Could you check a few things on this model? Use its own coordinates, in mm. A direction names the side the tool comes from. Round coordinates to 2 decimals unless told otherwise and drop trailing zeros. Write each loop counter-clockwise with the first axis right and the second up, starting at its lowest first coordinate (ties: lowest second). Pieces come first, ordered by that corner, then holes. Notation, with made-up numbers: (-35.75, 28.5) -> (9.25, 28.5) arc R14 cw to (9.25, 44.5) -> close; hole circle Ø6 at (-5.75, 34.25). An arc over 180 degrees is marked (long way). Answer in a Markdown table with one row per item.
from build123d import *

# Parameters (mm, degrees)
BOSS_EXTRUDE1_DEPTH      = 1.5
BOSS_EXTRUDE1_DEPTH_BACK = 1.5
SKETCH1_R                = 5
SKETCH1_R_2              = 2
FILLET1_R                = 100
SKETCH2_R                = 1.5
CUT_EXTRUDE1_DEPTH       = 10


with BuildPart() as part:
    # Sketch1 → Boss-Extrude1 (new, two sides: drawn at the far end of the back side and taken through both)
    with BuildSketch(Plane(origin=(0, 0, 0), x_dir=(1, 0, 0), z_dir=(0, 1, 0)).offset(-BOSS_EXTRUDE1_DEPTH_BACK)):
        with BuildLine():
            Line((0, 15), (-139.784941349, 43.225909045))
            Line((-139.784941349, 43.225909045), (-351.875415017, 29.941322925))
            ThreePointArc((-351.875415017, 29.941322925), (-378.412739548, -9.628926804), (-333.285739517, -24.912516864))
            Line((-333.285739517, -24.912516864), (-287.823465989, 5.588948968))
            Line((-287.823465989, 5.588948968), (-138.053278996, 13.889014505))
            Line((-138.053278996, 13.889014505), (-5.919683, -13.782501703))
            Line((-5.919683, -13.782501703), (0, -15))
            Line((0, -15), (40, -15))
            ThreePointArc((40, -15), (55, 0), (40, 15))
            Line((40, 15), (0, 15))
        make_face()
        with Locations(Location((0, 0, 0), (0, 0, 270))):
            Circle(SKETCH1_R, mode=Mode.SUBTRACT)
        with Locations(Location((40, 0, 0), (0, 0, 270))):
            Circle(SKETCH1_R_2, mode=Mode.SUBTRACT)
    extrude(amount=BOSS_EXTRUDE1_DEPTH + BOSS_EXTRUDE1_DEPTH_BACK)

    # Fillet1
    fillet1_edges = [part.edges().sort_by_distance(p)[0] for p in [
        (0, 0, -15),
        (-139.784941349, 0, -43.225909045),
        (-138.053278996, 0, -13.889014505),
        (-287.823465989, 0, -5.588948968),
        (0, 0, 15),
    ]]
    fillet(fillet1_edges, radius=FILLET1_R)

    # Sketch2 → Cut-Extrude1 (cut)
    with BuildSketch(Plane(origin=(0, 1.5, 0), x_dir=(1, 0, 0), z_dir=(0, 1, 0))):
        with Locations(Location((-147.336246923, 28.050603479, 0), (0, 0, 270))):
            Circle(SKETCH2_R)
        with Locations(Location((-130.791911053, 26.905656844, 0), (0, 0, 270))):
            Circle(SKETCH2_R)
        with Locations(Location((-364.746711272, 9.415773639, 0), (0, 0, 270))):
            Circle(SKETCH2_R)
        with Locations(Location((-348.032450789, -15.496743225, 0), (0, 0, 270))):
            Circle(SKETCH2_R)
    extrude(amount=-CUT_EXTRUDE1_DEPTH, mode=Mode.SUBTRACT)


solid = part.part
1) Imagine slicing it at C-C, the plane x = -238. Please give me the cut outline in (y, z).
Findings:
| item | result |
|---|---|
| outline | (-1.5, -37.07) -> (1.5, -37.07) -> (1.5, -8.35) -> (-1.5, -8.35) -> close |
2) Imagine slicing it at B-B, the plane y = -1. Count the separate pieces of the cut face and the enclosed holes in it, plus the area to 3 significant figures.
Findings:
| item | result |
|---|---|
| separate pieces | 1 |
| enclosed holes | 6 |
| area | 14,200 mm^2 |
3) Imagine slicing it at A-A, the plane x = -78.5. Please give me the cut outline in (y, z), plus the area to 3 significant figures.
Findings:
| item | result |
|---|---|
| outline | (-1.5, -30.85) -> (1.5, -30.85) -> (1.5, -1.42) -> (-1.5, -1.42) -> close |
| area | 88.3 mm^2 |
4) Please list where these lines run through material, in increasing order: line 1 (Z direction, x = 9, y = 0.7); line 2 (Z direction, x = 2.5, y = -0.1); line 3 (Z direction, x = -150.5, y = -0.7).
Findings:
| item | result |
|---|---|
| line 1 | z = -15 to 14.99 |
| line 2 | z = -15.28 to -4.33, 4.33 to 14.7 |
| line 3 | z = -42.53 to -13.2 |
5) Thinking about a two-plate mould opening in X: for faces 3 (the face through (-166, -1.5, -15)), 4 (the face through (-287.005, 0.021, -1.965)), 5 (the face through (-378.65, -0.02, 8.9)), which applies, +X half, -X half, draft (parallel to the pull), parting line (faces both ways), or undercut?
Findings:
| item | result |
|---|---|
| face 3 | draft |
| face 4 | undercut |
| face 5 | parting line |
6) For faces 1 (the face through (-4.88, -0.02, -1.08)), 2 (the face through (-68.511, -0.021, 0.675)), which set-ups out of +Z, -Z, +X, -X, +Y, -Y let a thin tool reach every point of the face, with its end or its side?
Findings:
| item | result |
|---|---|
| face 1 | +Y, -Y |
| face 2 | +Z, +Y, -Y |
7) For pin 1 (3.5 mm diameter, centred on x = -147.34, z = -28.05, fed in from +Y); pin 2 (0.9 mm diameter, centred on x = 22, y = 0.5, fed in from +Z); pin 3 (1.5 mm diameter, centred on y = -1, z = 11, fed in from +X); pin 4 (1.5 mm diameter, centred on x = 29.5, y = -0.5, fed in from -Z), each with a flat end and sliding along its axis, tell me the tip position at first contact or that it passes through.
Findings:
| item | result |
|---|---|
| pin 1 | stops at y = 1.5 |
| pin 2 | stops at z = 15 |
| pin 3 | stops at x = 50.95 |
| pin 4 | stops at z = -15 |
